from build123d import *

# Parameters (mm, degrees)
SKETCH1_R               = 28
SKETCH1_R_2             = 18
BOSS_EXTRUDE1_DEPTH     = 10
SKETCH5_R               = 28
SKETCH5_R_2             = 18
BOSS_EXTRUDE6_DEPTH     = 10
SKETCH6_R               = 25
SKETCH6_R_2             = 18
BOSS_EXTRUDE7_DEPTH     = 4
SKETCH7_R               = 1
CUT_EXTRUDE1_DEPTH      = 24
SKETCH8_W               = 56
SKETCH8_H               = 40
BOSS_EXTRUDE8_DEPTH     = 29.5
SKETCH9_W               = 25
SKETCH9_H               = 12.5
CUT_EXTRUDE2_DEPTH      = 45
SKETCH10_W              = 12
SKETCH10_H              = 17
CUT_EXTRUDE3_DEPTH      = 27
CUT_EXTRUDE4_DEPTH      = 42
CUT_EXTRUDE4_DEPTH_BACK = 16
CUT_EXTRUDE5_DEPTH      = 40
SKETCH14_R              = 1.5
CUT_EXTRUDE6_DEPTH      = 10


with BuildPart() as part:
    # Sketch1 → Boss-Extrude1 (new body)
    # profile 1 of 2: a face of its own
    with BuildSketch(Plane.XY):
        Circle(SKETCH1_R)
        Circle(SKETCH1_R_2, mode=Mode.SUBTRACT)
    # profile 2 of 2: a face of its own
    with BuildSketch(Plane.XY):
        with BuildLine():
            Line((-28, 80), (28, 80))
            Line((28, 80), (28, 0))
            ThreePointArc((28, 0), (0, 28), (-28, 0))
            Line((-28, 0), (-28, 80))
        make_face()
    extrude(amount=BOSS_EXTRUDE1_DEPTH)

    # Sketch5 → Boss-Extrude6 (add)
    with BuildSketch(Plane.XY.offset(10)):
        Circle(SKETCH5_R)
        Circle(SKETCH5_R_2, mode=Mode.SUBTRACT)
    extrude(amount=BOSS_EXTRUDE6_DEPTH)

    # Sketch6 → Boss-Extrude7 (add)
    with BuildSketch(Plane.XY.offset(20)):
        Circle(SKETCH6_R)
        Circle(SKETCH6_R_2, mode=Mode.SUBTRACT)
    extrude(amount=BOSS_EXTRUDE7_DEPTH)

    # Sketch7 → Cut-Extrude1 (cut)
    with BuildSketch(Plane.XY.offset(24)):
        with Locations((-10.75, 18.619546181)):
            Circle(SKETCH7_R)
        with Locations((10.75, 18.619546181)):
            Circle(SKETCH7_R)
        with Locations((21.5, 0)):
            Circle(SKETCH7_R)
        with Locations((10.75, -18.619546181)):
            Circle(SKETCH7_R)
        with Locations((-10.75, -18.619546181)):
            Circle(SKETCH7_R)
        with Locations((-21.5, 0)):
            Circle(SKETCH7_R)
    extrude(amount=-CUT_EXTRUDE1_DEPTH, mode=Mode.SUBTRACT)

    # Sketch8 → Boss-Extrude8 (add)
    with BuildSketch(Plane.XY.offset(10)):
        with Locations((0, 60)):
            Rectangle(SKETCH8_W, SKETCH8_H)
    extrude(amount=BOSS_EXTRUDE8_DEPTH)

    # Sketch9 → Cut-Extrude2 (cut)
    with BuildSketch(Plane(origin=(0, 80, 0), x_dir=(1, 0, 0), z_dir=(0, 1, 0))):
        with Locations((0, -33.25)):
            Rectangle(SKETCH9_W, SKETCH9_H)
    extrude(amount=-CUT_EXTRUDE2_DEPTH, mode=Mode.SUBTRACT)

    # Sketch10 → Cut-Extrude3 (cut)
    with BuildSketch(Plane(origin=(0, 80, 0), x_dir=(1, 0, 0), z_dir=(0, 1, 0))):
        with Locations((11, -8.5)):
            Rectangle(SKETCH10_W, SKETCH10_H)
        with Locations((-11, -8.5)):
            Rectangle(SKETCH10_W, SKETCH10_H)
    extrude(amount=-CUT_EXTRUDE3_DEPTH, mode=Mode.SUBTRACT)

    # Sketch11 → Cut-Extrude4 (cut, two sides: drawn at the far end of the back side and taken through both)
    with BuildSketch(Plane.ZY.offset(-17).offset(-CUT_EXTRUDE4_DEPTH_BACK)):
        Polygon((0, 53), (17, 80), (0, 80), align=None)
    extrude(amount=CUT_EXTRUDE4_DEPTH + CUT_EXTRUDE4_DEPTH_BACK, mode=Mode.SUBTRACT)

    # Sketch13 → Cut-Extrude5 (cut)
    with BuildSketch(Plane(origin=(0, 0, 0), x_dir=(-1, 0, 0), z_dir=(0, 0, -1))):
        Polygon((28, 80), (28, 0), (23, 80), align=None)
    cut_extrude5 = extrude(amount=-CUT_EXTRUDE5_DEPTH, mode=Mode.SUBTRACT)

    # Mirror1: Cut-Extrude5 across plane
    add(cut_extrude5.mirror(Plane(origin=(0, 0, 0), x_dir=(0, 0, 1), z_dir=(1, 0, 0))), mode=Mode.SUBTRACT)

    # Sketch14 → Cut-Extrude6 (cut)
    with BuildSketch(Plane(origin=(0, 0, 17), x_dir=(-1, 0, 0), z_dir=(0, 0, -1))):
        with Locations((-9, 70)):
            Circle(SKETCH14_R)
        with Locations((-9, 58)):
            Circle(SKETCH14_R)
        with Locations((9, 70)):
            Circle(SKETCH14_R)
        with Locations((9, 58)):
            Circle(SKETCH14_R)
    extrude(amount=-CUT_EXTRUDE6_DEPTH, mode=Mode.SUBTRACT)


solid = part.part
Source: CAD feature listing. Evaluate the final solid. Frame: model axes, mm. A direction names the side the tool comes from. Round coordinates to 2 decimals unless told otherwise and drop trailing zeros. Loops run counter-clockwise (first coordinate to the right, second up) from the corner with the lowest first, then second, coordinate; pieces in that order, holes last. Notation, with made-up numbers: (24.5, -39.5) - (61.5, -39.5) arc R16 ccw to (61.5, -11.5) - close; hole circle Ø8 at (72, 14.5). An arc over 180 degrees is marked (long way). Write item = value, one per line. Start each with the question number.
(1) Pull-direction query (Y, two-part tool) for faces 4 (the face through (19, 60, 39.5)), 5 (the face through (0, 30, 10)), 6 (the face through (-0.616, -27.993, 9.86)); classes: +Y half, -Y half, draft (parallel to the pull), parting line (faces both ways), or undercut.
(2) Ray query, line 1 along Y through (x, z) = (10.75, 6.5); line 2 along Z through (x, y) = (-17, 29); line 3 along X through (y, z) = (63, 13.5). Return the intervals inside material, ascending. Write a range as from..to.
(3) Section query C-C, the plane y = 70. Output: boundary loops of the cut face in (x, z) (3 decimals), plus the area to 3 significant figures.
(4) Pin query (flat end, axial travel): pin 1 (2.5 mm diameter, centred on x = -9, y = 70, fed in from -Z); pin 2 (5 mm diameter, centred on y = 70, z = 9, fed in from +X); pin 3 (10 mm diameter, centred on y = 50.5, z = 36.5, fed in from +X); pin 4 (3 mm diameter, centred on x = -21.5, y = 0, fed in from +Z). Return the tip coordinate at first contact, or that it passes through.
(5) Set-up query: faces 1 (the face through (17, 61, 12)), 2 (the face through (-10.967, 17.643, 12.168)), 3 (the face through (-11, 23, 20)). Return all of +Z, -Z, +X, -X, +Y, -Y with unobstructed straight access to the full face (end or side cutting, diameter ignored); none if empty.
(6) Section query D-D, the plane y = 13. Output: boundary loops of the cut face in (x, z), plus the area to 3 significant figures.
(7) Section query B-B, the plane z = 12.5. State how many separate pieces and enclosed holes the cut face has, plus the area to 3 significant figures.
(8) Section query A-A, the plane x = 0. Output: boundary loops of the cut face in (y, z), plus the area to 3 significant figures.
Conclusion:
q1.face_4 = draft
q1.face_5 = undercut
q1.face_6 = -Y half
q2.line_1 = -25.85..-19.62, -17.62..-14.44, 14.44..17.62, 19.62..53
q2.line_2 = 0..10
q2.line_3 = -24.06..-17, -5..5, 17..24.06
q3.outline = (-23.625, 10.704) - (-17, 10.704) - (-17, 17) - (-10.5, 17) - (-10.5, 27) - (-12.5, 27) - (-12.5, 39.5) - (-23.625, 39.5) - close; (-7.5, 17) - (-5, 17) - (-5, 10.704) - (5, 10.704) - (5, 17) - (7.5, 17) - (7.5, 27) - (-7.5, 27) - close; (10.5, 17) - (17, 17) - (17, 10.704) - (23.625, 10.704) - (23.625, 39.5) - (12.5, 39.5) - (12.5, 27) - (10.5, 27) - close
q3.area = 837 mm2
q4.pin_1 = through
q4.pin_2 = 23.78
q4.pin_3 = 25.16
q4.pin_4 = 24
q5.face_1 = -Z, +Y
q5.face_2 = +Z, -Z
q5.face_3 = +Z
q6.outline = (-27.19, 0) - (-12.45, 0) - (-12.45, 24) - (-21.35, 24) - (-21.35, 20) - (-24.8, 20) - (-24.8, 10) - (-27.19, 10) - close; (12.45, 0) - (27.19, 0) - (27.19, 10) - (24.8, 10) - (24.8, 20) - (21.35, 20) - (21.35, 24) - (12.45, 24) - close
q6.area = 613 mm2
q7.separate_pieces = 2
q7.enclosed_holes = 7
q7.area = 2,560 mm2
q8.outline = (-28, 0) - (-18, 0) - (-18, 24) - (-25, 24) - (-25, 20) - (-28, 20) - close; (18, 0) - (53, 0) - (80, 17) - (80, 27) - (40, 27) - (40, 10) - (28, 10) - (28, 20) - (25, 20) - (25, 24) - (18, 24) - close
q8.area = 1,430 mm2
